```python
from build123d import *

# Parameters (mm, degrees)
SKETCH1_W           = 146.05
SKETCH1_H           = 146.05
SKETCH1_R           = 6.35
SKETCH1_R_2         = 19.05
SKETCH1_R_3         = 3.175
SKETCH1_W_2         = 6.604
SKETCH1_H_2         = 19.05
BOSS_EXTRUDE1_DEPTH = 3.175
FILLET1_R           = 6.35


with BuildPart() as part:
    # Sketch1 → Boss-Extrude1 (new body, symmetric)
    with BuildSketch(Plane.XY):
        with Locations((-9.525, 0)):
            Rectangle(SKETCH1_W, SKETCH1_H)
        with Locations((50.8, 60.325)):
            Circle(SKETCH1_R, mode=Mode.SUBTRACT)
        with Locations((50.8, -60.325)):
            Circle(SKETCH1_R, mode=Mode.SUBTRACT)
        Circle(SKETCH1_R_2, mode=Mode.SUBTRACT)
        with Locations((0, 45)):
            Circle(SKETCH1_R_3, mode=Mode.SUBTRACT)
        with Locations((0, -45)):
            Circle(SKETCH1_R_3, mode=Mode.SUBTRACT)
        with Locations((-69.85, 60.325)):
            Circle(SKETCH1_R, mode=Mode.SUBTRACT)
        with Locations((-69.85, -60.325)):
            Circle(SKETCH1_R, mode=Mode.SUBTRACT)
        with Locations((-55.88, 0)):
            Rectangle(SKETCH1_W_2, SKETCH1_H_2, mode=Mode.SUBTRACT)
        with Locations((-55.88, 36.5125)):
            Rectangle(SKETCH1_W_2, SKETCH1_H_2, mode=Mode.SUBTRACT)
        with Locations((-55.88, -36.5125)):
            Rectangle(SKETCH1_W_2, SKETCH1_H_2, mode=Mode.SUBTRACT)
    extrude(amount=BOSS_EXTRUDE1_DEPTH, both=True)

    # Fillet1
    fillet1_edges = [part.edges().sort_by_distance(p)[0] for p in [
        (-82.55, 73.025, 0),
        (63.5, 73.025, 0),
        (63.5, -73.025, 0),
        (-82.55, -73.025, 0),
    ]]
    fillet(fillet1_edges, radius=FILLET1_R)


solid = part.part
```
The listing builds one solid part. Answer for the finished solid, in the listing's coordinates (mm). A direction names the side the tool comes from. Coordinates: 2 decimals unless noted, no trailing zeros. Loops run counter-clockwise (first coordinate to the right, second up) from the corner with the lowest first, then second, coordinate; pieces in that order, holes last. Notation, with made-up numbers: (18, 60) -> (65, 60) arc R16 cw to (65, 76) -> close; hole circle Ø4 at (-27.75, 56.5). An arc over 180 degrees is marked (long way). Return JSON: item names as keys, results as strings. Group by question number.
(1) A cutting plane is placed at C-C on x = 0. Write down the section's boundary in (y, z) (3 decimals).
(2) A cutting plane is placed at A-A on y = 0. Write down the section's boundary in (x, z) (3 decimals), and give its area (3 significant figures).
(3) Find the intervals of material crossed by probe 1 along X at (y, z) = (-60.5, -1.25); probe 2 along Y at (x, z) = (-69.85, -2) (3 decimals); probe 3 along X at (y, z) = (31.5, 2.25), in increasing order. Write a range as from..to.
(4) Determine the mould class of faces 3 (the flat face through (-10, 73.025, 0)), 4 (the cylindrical face through (61.689, 71.115, -0.044)), 5 (the flat face through (-59.182, -37, 0)), 6 (the cylindrical face through (-80.739, 71.115, -0.044)) for opening direction X: released by +X, released by -X, zero draft, split by the parting line, or undercut.
(5) Given pin 1 Ø16.5 at (x, y) = (-69.85, -60.325) entering from +Z (3 decimals), flat-ended and moving along its own axis, determine where the tip first touches the part or whether it passes through.
(6) A cutting plane is placed at B-B on x = -69.85. Write down the section's boundary in (y, z) (3 decimals).
(7) A cutting plane is placed at D-D on z = -0.25. Count the separate pieces of the cut face and the enclosed holes in it, and give its area (3 significant figures).
(8) Which of the six approach directions +Z, -Z, +X, -X, +Y, -Y give full straight-line access (tool end or side, diameter ignored) to faces 1 (the flat face through (-10, -73.025, 0)), 2 (the flat face through (-59.182, 36, 0))?
The answers:
{
 "1": {"outline": "(-73.025, -3.175) -> (-48.175, -3.175) -> (-48.175, 3.175) -> (-73.025, 3.175) -> close; (-41.825, -3.175) -> (-19.05, -3.175) -> (-19.05, 3.175) -> (-41.825, 3.175) -> close; (19.05, -3.175) -> (41.825, -3.175) -> (41.825, 3.175) -> (19.05, 3.175) -> close; (48.175, -3.175) -> (73.025, -3.175) -> (73.025, 3.175) -> (48.175, 3.175) -> close"},
 "2": {"outline": "(-82.55, -3.175) -> (-59.182, -3.175) -> (-59.182, 3.175) -> (-82.55, 3.175) -> close; (-52.578, -3.175) -> (-19.05, -3.175) -> (-19.05, 3.175) -> (-52.578, 3.175) -> close; (19.05, -3.175) -> (63.5, -3.175) -> (63.5, 3.175) -> (19.05, 3.175) -> close", "area": "644 mm^2"},
 "3": {"probe 1": "x = -82.55..-76.2, -63.5..44.45, 57.15..63.5", "probe 2": "y = -73.025..-66.675, -53.975..53.975, 66.675..73.025", "probe 3": "x = -82.55..-59.18, -52.58..63.5"},
 "4": {"face 3": "zero draft", "face 4": "released by +X", "face 5": "undercut", "face 6": "released by -X"},
 "5": {"pin 1": "stops at z = 3.175"},
 "6": {"outline": "(-73.025, -3.175) -> (-66.675, -3.175) -> (-66.675, 3.175) -> (-73.025, 3.175) -> close; (-53.975, -3.175) -> (53.975, -3.175) -> (53.975, 3.175) -> (-53.975, 3.175) -> close; (66.675, -3.175) -> (73.025, -3.175) -> (73.025, 3.175) -> (66.675, 3.175) -> close"},
 "7": {"separate pieces": "1", "enclosed holes": "10", "area": "19,200 mm^2"},
 "8": {"face 1": "+Z, -Z, +X, -X, -Y", "face 2": "+Z, -Z"}
}
